Drawing for the job (mm, zero at the part's lowest x, y, z). A direction names the side the tool comes from. Give positions to 0.01 mm unless a question says otherwise; leave off trailing zeros. Loops run counter-clockwise (first coordinate to the right, second up) from the corner with the lowest first, then second, coordinate; pieces in that order, holes last. Notation, with made-up numbers: M 49,11 L 77,11 A15 cw 77,35 Z; hole C -10,5.5 d8. An arc over 180 degrees is marked long. Use CSV: the item, a comma, the result in double quotes. Start each with the question number.
(1) Slice it at D-D on x = 1065.5. List the corners of the cut face in (y, z), and give its area (3 significant figures).
(2) Slice it at A-A on x = 1898.5. List the corners of the cut face in (y, z).
(3) Slice it at C-C on y = 207. List the corners of the cut face in (x, z) (1 decimal), and give its area (3 significant figures).
(4) Flat gauge pin, fed straight in: P1, Ø12, axis at y = 297, z = 709.5, coming from the +X side. Where does the tip first touch, or does it go through?
(5) Wall check: line 1 along Y through (x, z) = (466, 892); line 2 along Z through (x, y) = (1903, 363). Give the ranges that are in metal, low to high. Write a range as from..to.
(6) Tool access for the marked faces 1, 2 and 3: list every direction of +Z, -Z, +X, -X, +Y, -Y with a clear straight run to the whole face (end or side of a thin tool).
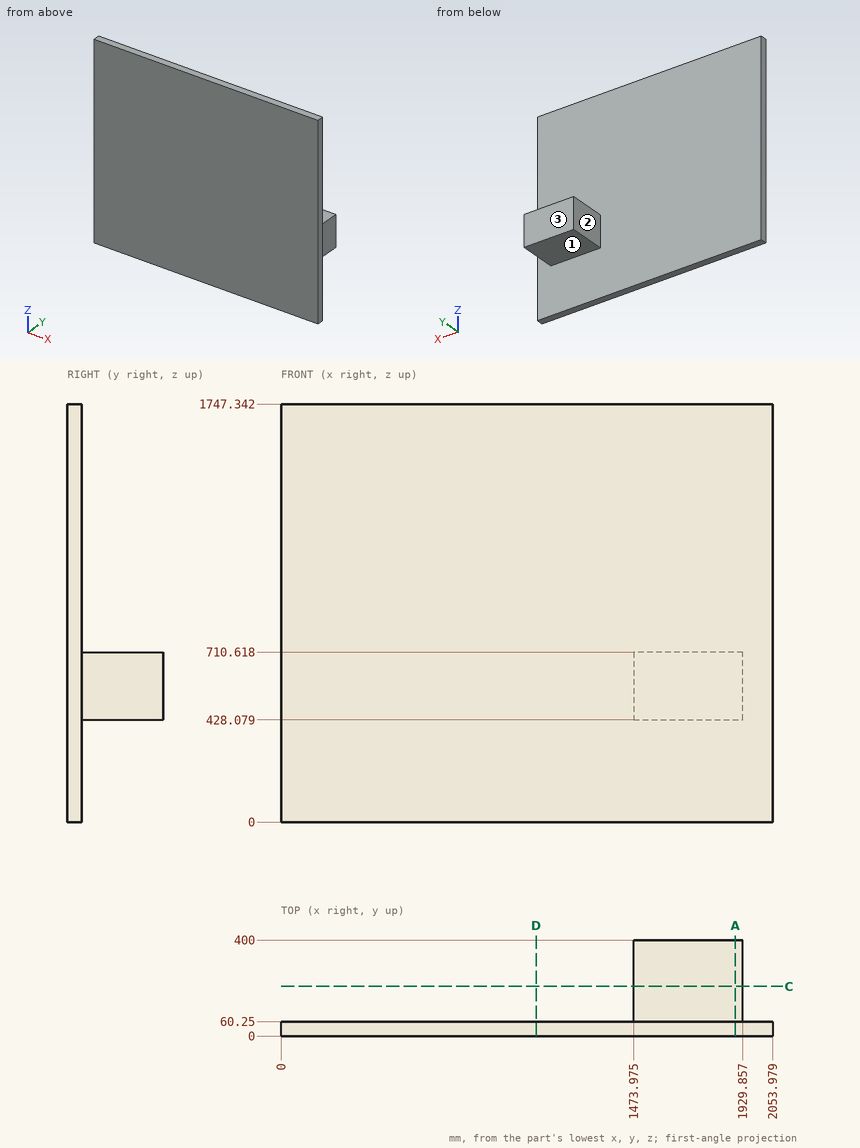
Reply:
1,outline,"M 0,0 L 60.25,0 L 60.25,1747.34 L 0,1747.34 Z"
1,area,"105,000 mm^2"
2,outline,"M 0,0 L 60.25,0 L 60.25,428.08 L 400,428.08 L 400,710.62 L 60.25,710.62 L 60.25,1747.34 L 0,1747.34 Z"
3,outline,"M 1474,428.1 L 1929.9,428.1 L 1929.9,710.6 L 1474,710.6 Z"
3,area,"129,000 mm^2"
4,P1,"stops at x = 1929.86"
5,line 1,"y = 0..60.25"
5,line 2,"z = 428.08..710.62"
6,face 1,"-Z, +X, -X, +Y"
6,face 2,"+Z, -Z, -X, +Y"
6,face 3,"+Z, -Z, +X, -X, +Y"
